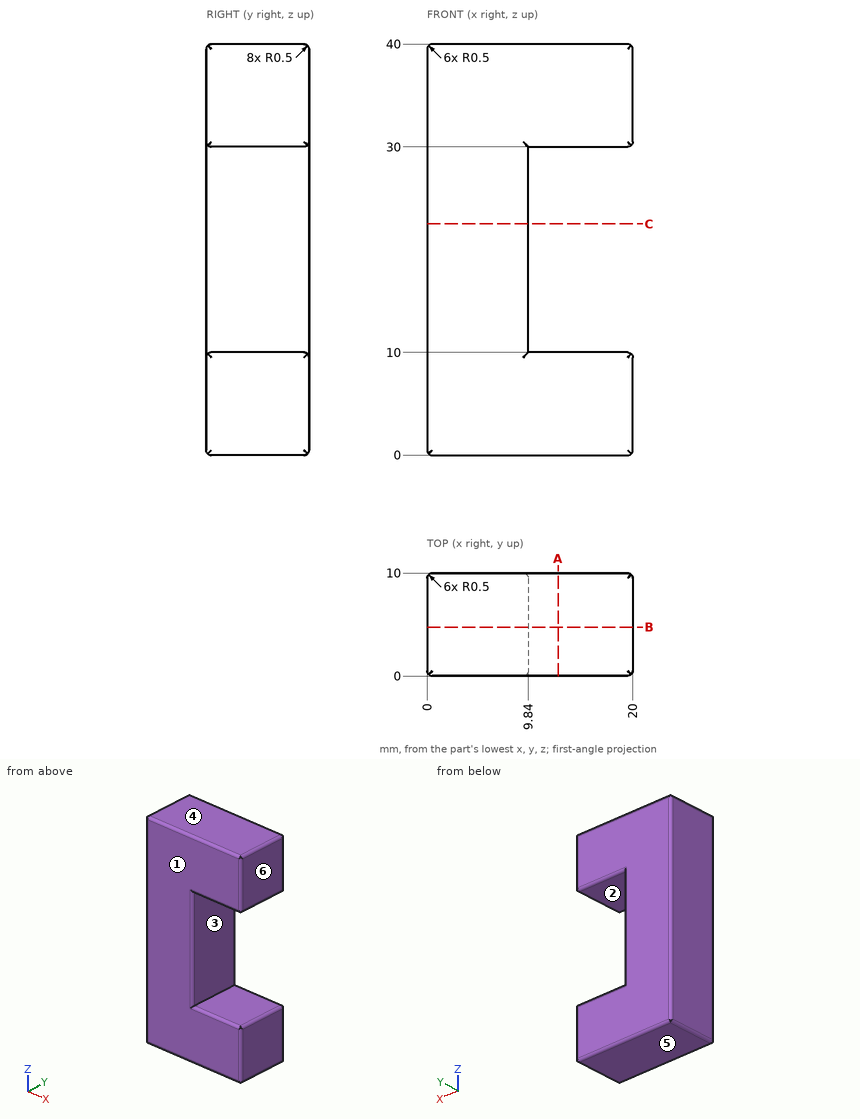
For this review, use the dimensioned drawing (mm, ordinates from the lowest corner) and the shaded views. A direction names the side the tool comes from. Round coordinates to 2 decimals unless told otherwise and drop trailing zeros. Write each loop counter-clockwise with the first axis right and the second up, starting at its lowest first coordinate (ties: lowest second). Pieces come first, ordered by that corner, then holes. Notation, with made-up numbers: (-38.75, 0.25) - (17.25, 0.25) arc R20 cw to (17.25, 27.25) - close; hole circle Ø11 at (77, 69.5). An arc over 180 degrees is marked (long way). Answer as CSV lines item,"result". Start each with the question number.
(1) Draft analysis for pull direction Z (two halves, no side actions). For the marked faces 3, 4, 5 and 6, state which applies: pulls with the +Z half, pulls with the -Z half, needs draft (parallel to the pull), parting line crosses it, or undercut.
(2) For pin 1 Ø2.5 at (y, z) = (5.5, 17) entering from +X; pin 2 Ø10 at (x, z) = (15.5, 22.5) entering from +Y, all flat-tipped, find the tip position at first contact; note any pin that passes through.
(3) We need section B-B on y = 4.75. State the section outline as (x, z) points.
(4) We need section C-C on z = 22.5. State the section outline as (x, y) points.
(5) To check wall thickness, follow line 1 (Z direction, x = 12, y = 2.5); line 2 (X direction, y = 2.75, z = 15). State the ranges of each line that lie inside material, in increasing order.
(6) For the marked faces 1 and 2, list the 3-axis set-ups (+Z, -Z, +X, -X, +Y, -Y) from which the entire face can be reached by the end or side of a thin tool; tool diameter is ignored.
(7) We need section A-A on x = 12.75. State the section outline as (y, z) points, plus the area to 3 significant figures.
Worked answers:
1,face 3,"undercut"
1,face 4,"pulls with the +Z half"
1,face 5,"pulls with the -Z half"
1,face 6,"needs draft"
2,pin 1,"x = 9.84"
2,pin 2,"through"
3,outline,"(0, 0.5) arc R0.5 ccw to (0.5, 0) - (19.5, 0) arc R0.5 ccw to (20, 0.5) - (20, 9.5) arc R0.5 ccw to (19.5, 10) - (9.84, 10) - (9.84, 30) - (19.5, 30) arc R0.5 ccw to (20, 30.5) - (20, 39.5) arc R0.5 ccw to (19.5, 40) - (0.5, 40) arc R0.5 ccw to (0, 39.5) - close"
4,outline,"(0, 0.5) arc R0.5 ccw to (0.5, 0) - (9.34, 0) arc R0.5 ccw to (9.84, 0.5) - (9.84, 9.5) arc R0.5 ccw to (9.34, 10) - (0.5, 10) arc R0.5 ccw to (0, 9.5) - close"
5,line 1,"0 to 10, 30 to 40"
5,line 2,"0 to 9.84"
6,face 1,"+Z, -Z, +X, -X, -Y"
6,face 2,"+X, +Y, -Y"
7,outline,"(0, 0.5) arc R0.5 ccw to (0.5, 0) - (9.5, 0) arc R0.5 ccw to (10, 0.5) - (10, 9.5) arc R0.5 ccw to (9.5, 10) - (0.5, 10) arc R0.5 ccw to (0, 9.5) - close; (0, 30.5) arc R0.5 ccw to (0.5, 30) - (9.5, 30) arc R0.5 ccw to (10, 30.5) - (10, 39.5) arc R0.5 ccw to (9.5, 40) - (0.5, 40) arc R0.5 ccw to (0, 39.5) - close"
7,area,"200 mm²"
